from build123d import *

# Parameters (mm, degrees)
BOX_W          = 70
BOX_H          = 14
BOX_DEPTH      = 2.5
CYLINDER_R     = 2
CYLINDER_DEPTH = 3.5


with BuildPart() as part:
    # Box → Box (join)
    with BuildSketch(Plane.XY):
        with Locations((35, 7)):
            Rectangle(BOX_W, BOX_H)
    extrude(amount=BOX_DEPTH)

    # Cylinder → Cylinder (cut)
    with BuildSketch(Plane(origin=(35, 7, -1), x_dir=(1, 0, 0), z_dir=(0, 0, 1))):
        Circle(CYLINDER_R)
    extrude(amount=CYLINDER_DEPTH, mode=Mode.SUBTRACT)


solid = part.part
Input: part model. Units: mm. Frame: model coordinates. Give positions to 0.01 mm unless a question says otherwise; leave off trailing zeros. Write each loop counter-clockwise with the first axis right and the second up, starting at its lowest first coordinate (ties: lowest second). Pieces come first, ordered by that corner, then holes. Notation, with made-up numbers: M -39,-15 L -7,-15 A9 cw -7,0 Z; hole C 67,88.5 d4. An arc over 180 degrees is marked long. Write item = value, one per line. Start each with the question number.
1) Draft query along X for faces 1 (the flat face through (35, 14, 1)), 2 (the flat face through (0, 7, 1)), 3 (the cylindrical face through (36.908, 7.601, 1.232)), 4 (the flat face through (70, 7, 1)). Return one class per face: +X half, -X half, draft (parallel to the pull), parting line (faces both ways), or undercut.
2) Cut plane A-A on y = 7. Return the cut outline in (x, z).
3) Cut plane B-B on x = 35. Return the cut outline in (y, z), then the cut area to 3 significant figures.
4) Material intervals for line 1 along Y through (x, z) = (35, 0.75); line 2 along X through (y, z) = (7, 1.2); line 3 along Y through (x, z) = (34, 1.3), sorted ascending. Write a range as [from, to].
Solved:
q1.face_1 = draft
q1.face_2 = -X half
q1.face_3 = undercut
q1.face_4 = +X half
q2.outline = M 0,0 L 33,0 L 33,2.5 L 0,2.5 Z; M 37,0 L 70,0 L 70,2.5 L 37,2.5 Z
q3.outline = M 0,0 L 5,0 L 5,2.5 L 0,2.5 Z; M 9,0 L 14,0 L 14,2.5 L 9,2.5 Z
q3.area = 25.0 mm2
q4.line_1 = [0, 5], [9, 14]
q4.line_2 = [0, 33], [37, 70]
q4.line_3 = [0, 5.27], [8.73, 14]
